```python
from build123d import *

# Parameters (mm, degrees)
F5_D            = 6.6
F5_DEPTH        = 15
F5_START        = 0.126815
F5_TIP          = 1.9828400428
F5_COPIES_COUNT = 3


# Not quite as in the source:
# - a pattern or mirror of a feature is missing from the dataset's text; its kind, count and spacing are read off the source's solid


with BuildPart() as f1:
    # F0 (on Front) → F1 (revolve)
    with BuildSketch(Plane.XZ):
        Polygon((0, 43), (0, 35), (37, 35), (37, 43), (16, 43), (16, 40), (8, 40), (8, 43), align=None)
    revolve(axis=Axis((12.3033272102, 0, 0), (1, 0, 0)))

    # F5
    # its depths count from where the whole tool has entered the part; down to there all is cleared
    with Locations(Plane.XY.offset(43).offset(-F5_START)):
        with Locations((32.0342332125, 0)):
            f5 = Hole(F5_D / 2, depth=F5_DEPTH)
            with Locations((0, 0, -(F5_DEPTH + F5_TIP / 2))):  # 118° drill point
                Cone(0, F5_D / 2, F5_TIP, mode=Mode.SUBTRACT)

    # F5_copies: F5 ×3 about axis
    f5_copies_axis = Axis((0, 0, 0), (1, 0, 0))
    for i in range(1, F5_COPIES_COUNT):
        add(f5.rotate(f5_copies_axis, i * 360 / F5_COPIES_COUNT), mode=Mode.SUBTRACT)


solid = f1.part
```
Here's how the part is built. I have some questions about the finished solid (model axes, mm). A direction names the side the tool comes from. Round coordinates to 2 decimals unless told otherwise and drop trailing zeros. Order: outer loops, then holes, each group sorted by start corner. A loop starts at its lowest first (then second) coordinate and runs counter-clockwise, first axis right, second up. Notation, with made-up numbers: (12, -22.75) -> (16, -22.75) arc R27 ccw to (16, 9.25) -> close; hole circle Ø7 at (25, 50). An arc over 180 degrees is marked (long way). Use a Markdown table: item, result. Add a question column.
(1) For pin 1 Ø1.5 at (x, z) = (28, 27) entering from -Y; pin 2 Ø2 at (x, y) = (14, -25.5) entering from +Z; pin 3 Ø4 at (x, z) = (13.5, 21) entering from +Y, each with a flat end and sliding along its axis, tell me the tip position at first contact or that it passes through.
(2) Suppose I cut it at C-C, the plane y = 11. Please give me the cut outline in (x, z), and give its area (3 significant figures).
(3) Suppose I cut it at D-D, the plane x = 31. Please give me the cut outline in (y, z), and give its area (3 significant figures).
(4) I need wall thicknesses on line 1 along X through (y, z) = (-20.5, 37); line 2 along Z through (x, y) = (26, 0). Which ranges of each line are inside material? Lowest first, please.
(5) If we mould it in two halves opening along Z, with no side actions, what happens to faces 1 (the face through (35.33, -33.73, -19.31)), 2 (the face through (3.944, -42.634, -5.598)), 3 (the face through (0, 35, 6))? For each: released by +Z, released by -Z, zero draft, split by the parting line, or undercut.
(6) Suppose I cut it at B-B, the plane z = 0. Please give me the cut outline in (x, y), and give its area (3 significant figures).
(7) Suppose I cut it at A-A, the plane y = 0. Please give me the cut outline in (x, z).
(8) For faces 4 (the face through (8, 38, -13)), 5 (the face through (19, 21, -28)), 6 (the face through (35.33, 0.15, 38.86)), which set-ups out of +Z, -Z, +X, -X, +Y, -Y let a thin tool reach every point of the face, with its end or its side?
Verdict:
| question | item | result |
|---|---|---|
| 1 | pin 1 | y = -34.06 |
| 1 | pin 2 | z = 31.62 |
| 1 | pin 3 | y = 35.2 |
| 2 | outline | (0, -41.57) -> (8, -41.57) -> (8, -38.46) -> (16, -38.46) -> (16, -41.57) -> (37, -41.57) -> (37, -33.23) -> (0, -33.23) -> close; (0, 33.23) -> (37, 33.23) -> (37, 41.57) -> (16, 41.57) -> (16, 38.46) -> (8, 38.46) -> (8, 41.57) -> (0, 41.57) -> close |
| 2 | area | 568 mm2 |
| 3 | outline | (-38.71, -18.73) -> (-31.76, -14.72) arc R35 cw to (-3.13, 34.86) -> (-3.13, 42.89) arc R43 ccw to start; (-35.57, -24.16) arc R43 ccw to (35.57, -24.16) -> (28.62, -20.14) arc R35 cw to (-28.62, -20.14) -> close; (3.13, 34.86) arc R35 cw to (31.76, -14.72) -> (38.71, -18.73) arc R43 ccw to (3.13, 42.89) -> close |
| 3 | area | 1,810 mm2 |
| 4 | line 1 | 0 to 8, 16 to 37 |
| 4 | line 2 | -43 to -35, 35 to 43 |
| 5 | face 1 | undercut |
| 5 | face 2 | split by the parting line |
| 5 | face 3 | zero draft |
| 6 | outline | (0, -43) -> (8, -43) -> (8, -40) -> (16, -40) -> (16, -43) -> (37, -43) -> (37, -35) -> (0, -35) -> close; (0, 35) -> (37, 35) -> (37, 43) -> (16, 43) -> (16, 40) -> (8, 40) -> (8, 43) -> (0, 43) -> close |
| 6 | area | 544 mm2 |
| 7 | outline | (0, -43) -> (8, -43) -> (8, -40) -> (16, -40) -> (16, -43) -> (37, -43) -> (37, -35) -> (0, -35) -> close; (0, 35) -> (28.73, 35) -> (28.73, 43) -> (16, 43) -> (16, 40) -> (8, 40) -> (8, 43) -> (0, 43) -> close; (35.33, 35) -> (37, 35) -> (37, 43) -> (35.33, 43) -> close |
| 8 | face 4 | none |
| 8 | face 5 | +X, -X |
| 8 | face 6 | +Z |
